Source: CAD feature listing. Evaluate the final solid. Frame: model axes, mm. Face numbers are marked on the shaded views. A direction names the side the tool comes from. Coordinates: 2 decimals unless noted, no trailing zeros. Write each loop counter-clockwise with the first axis right and the second up, starting at its lowest first coordinate (ties: lowest second). Pieces come first, ordered by that corner, then holes. Notation, with made-up numbers: (57, 22) - (110, 22) arc R16 cw to (110, 49) - close; hole circle Ø8 at (-13.75, 31.25). An arc over 180 degrees is marked (long way). One line per question, with ' | ' between items. Start each with the question number.
Q1. Line query: line 1 (Y direction, x = -8.5, z = -30.01); line 2 (Z direction, x = -1.75, y = 21); line 3 (Y direction, x = -2.25, z = -29). Output: solid intervals per line, ascending.
Q2. Access query for the marked faces 4 and 5. Directions: +Z, -Z, +X, -X, +Y, -Y. A direction counts if a zero-diameter tool reaches every point of the face in a straight line with its end or side. Return the directions, or none.
Q3. Cut plane C-C, the plane y = 25.5. Return loops of the section in (x, z) (3 decimals), plus the area to 3 significant figures.
Q4. Cut plane B-B, the plane y = 21.75. Return loops of the section in (x, z), plus the area to 3 significant figures.
Q5. Draft query along Y for the marked faces 1, 2 and 3. Return one class per face: +Y half, -Y half, draft (parallel to the pull), parting line (faces both ways), or undercut.
Q6. Cut plane D-D, the plane z = -10. Return loops of the section in (x, y).
Q7. Contact query for flat-ended pins moving along their axis: P1, Ø6.5, axis at x = -5.9, z = -30.01, coming from the -Y side; P2, Ø1, axis at y = 32.5, z = -8, coming from the +X side; P3, Ø3.5, axis at y = 5.75, z = -30.01, coming from the -X side; P4, Ø1.2, axis at x = -6, z = -21.5, coming from the +Y side. Output: stop coordinate, or through.
Q8. Cut plane A-A, the plane z = -30.01. Return loops of the section in (x, y) (3 decimals).
Autodesk Inventor part; units mm, degrees
ref_plane "YZ Plane" through (0, 0, 0) normal (1, 0, 0) x (0, 1, 0)
ref_plane "XZ Plane" through (0, 0, 0) normal (0, 1, 0) x (-1, 0, 0)
ref_plane "XY Plane" through (0, 0, 0) normal (0, 0, 1) x (1, 0, 0)
sketch "Sketch1" plane through (0, 0, 0) normal (0, 1, 0) x (-1, 0, 0)
  line L0 (0, 0) -> (11.8, 0)
  line L1 (11.8, 0) -> (11.8, -34)
  line L2 (11.8, -34) -> (0, -34)
  line L3 (0, -34) -> (0, 0)
  circle A0 centre (5.9, -30.01) radius 2.075
  dimension "d0" = 11.8
  dimension "d1" = 34
  dimension "d2" = 4.15
  dimension "d3" = 30.01
extrude "Extrusion1" add sketch "Sketch1" along normal blind 27.5
sketch "Sketch2" plane through (0, 27.5, 0) normal (0, 1, 0) x (1, 0, 0)
  circle A0 centre (-5.9, 6.01) radius 3.25
  line L0 (-11.8, 0) -> (0, 0)
  line L1 (0, 0) -> (0, 34)
  dimension "d6" = 6.5
  dimension "d7" = 6.01
  dimension "d8" = 5.9
extrude "Extrusion2" add sketch "Sketch2" along normal blind 5.7
sketch "Sketch3" plane through (-5.9, 33.2, -6.01) normal (0, 1, 0) x (1, 0, 0)
  line L0 (-4.85, -4.85) -> (4.85, -4.85)
  line L1 (4.85, -4.85) -> (4.85, 4.85)
  line L2 (4.85, 4.85) -> (-4.85, 4.85)
  line L3 (-4.85, 4.85) -> (-4.85, -4.85)
  line L4 (-4.85, -4.85) -> (4.85, 4.85) construction
  line L5 (4.85, -4.85) -> (-4.85, 4.85) construction
  point P0 (5.9, -6.01)
  point P1 (0, 0)
  dimension "d11" = 9.7
  dimension "d12" = 9.7
extrude "Extrusion3" add sketch "Sketch3" against normal blind 2
sketch "Sketch4" plane through (0, 0, 0) normal (0, -1, 0) x (1, 0, 0)
  circle A0 centre (-5.9, -6.01) radius 3.25
  circle A1 centre (-5.9, -6.01) radius 1.975
  point P0 (0, 0)
  dimension "d24" = 3.95
extrude "Extrusion4" add sketch "Sketch4" along normal blind 2 contours A1
sketch "Sketch5" plane through (0, 27.5, 0) normal (0, 1, 0) x (1, 0, 0)
  circle A0 centre (-5.9, 22.01) radius 1.975
  circle A1 centre (-5.9, 30.01) radius 2.075
  point P0 (0, 0)
  dimension "d27" = 3.95
  dimension "d28" = 8
extrude "Extrusion5" add sketch "Sketch5" along normal blind 2 contours A0
sketch "Sketch6" plane through (0, 0, 0) normal (0, -1, 0) x (1, 0, 0)
  circle A0 centre (-5.9, -22.01) radius 1.975
  circle A1 centre (-5.9, -22.01) radius 1.975
  point P0 (0, 0)
extrude "Extrusion6" add sketch "Sketch6" along normal blind 2
sketch "Sketch7" plane through (0, 0, 0) normal (1, 0, 0) x (0, 0, -1)
  circle A0 centre (30.01, 21.75) radius 2.2
  circle A1 centre (30.01, 5.75) radius 2.2
  line L0 (0, 27.5) -> (34, 27.5)
  line L1 (0, 0) -> (34, 0)
  line L2 (34, 0) -> (34, 27.5)
  dimension "d53" = 4.4
  dimension "d54" = 4.4
  dimension "d55" = 16
  dimension "d57" = 5.75
  dimension "d60" = 3.99
  dimension "d61" = 3.99
extrude "Extrusion7" cut sketch "Sketch7" against normal blind 17.25
properties part number "MS-1.5A Servo"
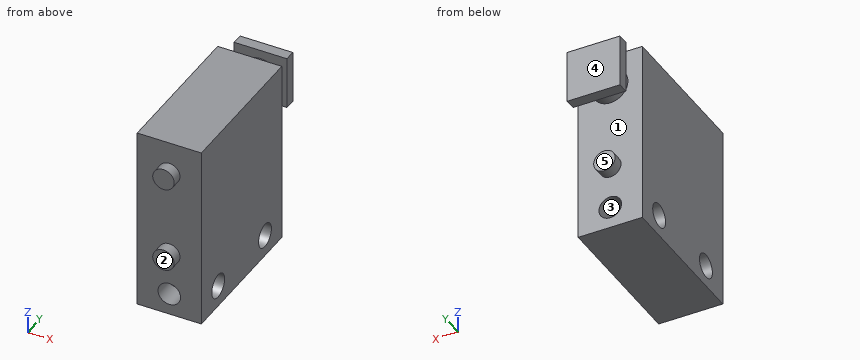
Reply:
1) line 1: y = 0 to 3.55, 7.95 to 19.55, 23.95 to 27.5 | line 2: z = -34 to -32.08, -27.94 to 0 | line 3: y = 0 to 3.8, 7.7 to 19.8, 23.7 to 27.5
2) face 4: +Z, -Z, +X, -X, +Y | face 5: -Z, +X, -X, +Y
3) outline: (-11.8, -34) - (0, -34) - (0, 0) - (-11.8, 0) - close; hole circle Ø4.15 at (-5.9, -30.01) | area: 388 mm^2
4) outline: (-11.8, -34) - (0, -34) - (0, -32.21) - (-11.8, -32.21) - close; (-11.8, -27.81) - (0, -27.81) - (0, 0) - (-11.8, 0) - close | area: 349 mm^2
5) face 1: undercut | face 2: -Y half | face 3: draft
6) outline: (-11.8, 0) - (0, 0) - (0, 27.5) - (-11.8, 27.5) - close; (-10.75, 31.2) - (-1.05, 31.2) - (-1.05, 33.2) - (-10.75, 33.2) - close
7) P1: stops at y = 0 | P2: stops at x = -1.05 | P3: passes through | P4: stops at y = 29.5
8) outline: (-11.8, 0) - (-7.975, 0) - (-7.975, 3.55) - (-11.8, 3.55) - close; (-11.8, 7.95) - (-7.975, 7.95) - (-7.975, 19.55) - (-11.8, 19.55) - close; (-11.8, 23.95) - (-7.975, 23.95) - (-7.975, 27.5) - (-11.8, 27.5) - close; (-3.825, 0) - (0, 0) - (0, 3.55) - (-3.825, 3.55) - close; (-3.825, 7.95) - (0, 7.95) - (0, 19.55) - (-3.825, 19.55) - close; (-3.825, 23.95) - (0, 23.95) - (0, 27.5) - (-3.825, 27.5) - close
